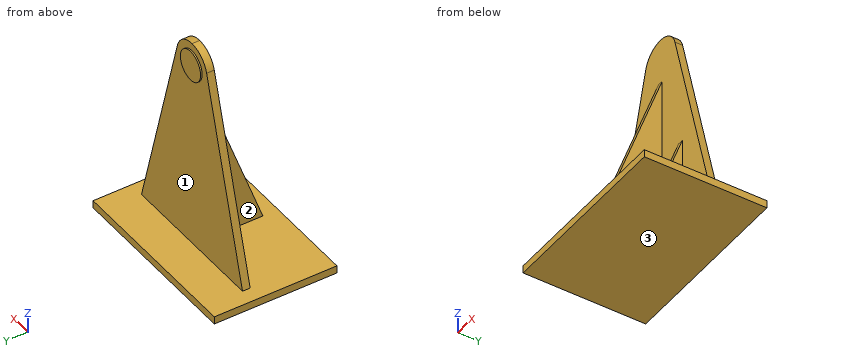
```python
from build123d import *

# Parameters (mm, degrees)
SKETCH1_W      = 152.4
SKETCH1_H      = 101.6
EXTRUDE1_DEPTH = 6.35
EXTRUDE2_DEPTH = 6.35
SKETCH4_R      = 12.7
EXTRUDE3_DEPTH = 1.27
EXTRUDE4_DEPTH = 2.38125
RIB4_REACH     = 218.366
SKETCH8_WALL_W = 509.057660384
SKETCH8_WALL_H = 4.7625


with BuildPart() as part:
    # Sketch1 → Extrude1 (new body)
    with BuildSketch(Plane.XY):
        Rectangle(SKETCH1_W, SKETCH1_H)
    extrude(amount=EXTRUDE1_DEPTH)

    # Sketch3 → Extrude2 (add)
    with BuildSketch(Plane(origin=(0, 19.05, 0), x_dir=(-1, 0, 0), z_dir=(0, 1, 0))):
        with BuildLine():
            Line((63.5, 6.35), (18.365629617, 170.160251847))
            ThreePointArc((18.365629617, 170.160251847), (11.54349822, 180.254212248), (0, 184.15))
            ThreePointArc((0, 184.15), (-11.54349822, 180.254212248), (-18.365629617, 170.160251847))
            Line((-18.365629617, 170.160251847), (-63.5, 6.35))
            Line((-63.5, 6.35), (63.5, 6.35))
        make_face()
    extrude(amount=-EXTRUDE2_DEPTH)

    # Sketch4 → Extrude3 (add)
    with BuildSketch(Plane(origin=(0, 19.05, 0), x_dir=(-1, 0, 0), z_dir=(0, 1, 0))):
        with Locations(Location((0, 165.1, 0), (0, 0, 270))):
            Circle(SKETCH4_R)
    extrude(amount=EXTRUDE3_DEPTH)

    # Sketch5 → Extrude4 (add, symmetric)
    with BuildSketch(Plane(origin=(0, 0, 0), x_dir=(0, 0, -1), z_dir=(1, 0, 0))):
        Polygon((-146.05, 12.7), (-6.35, -38.1), (-6.35, 12.7), align=None)
    extrude(amount=EXTRUDE4_DEPTH, both=True)

    # Sketch8 wall → Rib4 (add, up to next)
    with BuildSketch(Plane(origin=(25.4, 0, 41.275), x_dir=(0, -0.341743063087, -0.939793423488), z_dir=(0, 0.939793423488, -0.341743063087)), mode=Mode.PRIVATE) as rib4_sk1:
        Rectangle(SKETCH8_WALL_W, SKETCH8_WALL_H)
    rib4_tool1 = extrude(rib4_sk1.sketch, amount=RIB4_REACH, mode=Mode.PRIVATE) - part.part
    add(rib4_tool1.solids().sort_by_distance((25.4, 0, 41.275))[0])


solid = part.part
```
Verification items for the finished model (mm, model axes). Face numbers are marked on the shaded views. Round coordinates to 2 decimals unless told otherwise and drop trailing zeros. Order: outer loops, then holes, each group sorted by start corner. A loop starts at its lowest first (then second) coordinate and runs counter-clockwise, first axis right, second up.
1) Cross-section at C-C, the plane y = 32. Record the cut outline in (x, z).
Geometry says:
outline: (-76.2, 0) - (76.2, 0) - (76.2, 6.35) - (-76.2, 6.35) - close
2) Cross-section at D-D, the plane z = 38. Record the cut outline in (x, y).
Geometry says:
outline: (-54.78, 12.7) - (-2.38, 12.7) - (-2.38, -26.59) - (2.38, -26.59) - (2.38, 12.7) - (23.02, 12.7) - (23.02, -1.19) - (27.78, -1.19) - (27.78, 12.7) - (54.78, 12.7) - (54.78, 19.05) - (-54.78, 19.05) - close
3) Cross-section at A-A, the plane x = 43. Record the cut outline in (y, z), plus the area to 3 significant figures.
Geometry says:
outline: (-50.8, 0) - (50.8, 0) - (50.8, 6.35) - (19.05, 6.35) - (19.05, 80.75) - (12.7, 80.75) - (12.7, 6.35) - (-50.8, 6.35) - close
area: 1,120 mm2
4) Draft check along Z on the marked faces 1, 2 and 3. Enter one of: +Z half, -Z half, draft (parallel to the pull), parting line (faces both ways), or undercut.
Geometry says:
face 1: undercut
face 2: draft
face 3: -Z half
5) Material ranges on line 1 (Z direction, x = 58.5, y = -17.5); line 2 (Y direction, x = -31, z = 113); line 3 (X direction, y = -11, z = 64.5), recorded low to high.
Geometry says:
line 1: z = 0 to 6.35
line 2: y = 12.7 to 19.05
line 3: x = -2.38 to 2.38
6) Cross-section at B-B, the plane z = 131. Record the cut outline in (x, y).
Geometry says:
outline: (-29.16, 12.7) - (-2.38, 12.7) - (-2.38, 7.23) - (2.38, 7.23) - (2.38, 12.7) - (29.16, 12.7) - (29.16, 19.05) - (-29.16, 19.05) - close
7) Depth check by flat-ended pin: pin 1 (5 mm diameter, centred on x = -53, z = 40, fed in from -Y); pin 2 (8 mm diameter, centred on x = 57.5, y = 25.5, fed in from +Z); pin 3 (1 mm diameter, centred on x = -8.5, z = 62.5, fed in from +Y). Enter the tip coordinate at first touch or a pass-through.
Geometry says:
pin 1: stops at y = 12.7
pin 2: stops at z = 6.35
pin 3: stops at y = 19.05
